The model under review builds one solid part; all positions refer to its coordinate system, in mm. A direction names the side the tool comes from. Give positions to 0.01 mm unless a question says otherwise; leave off trailing zeros. Order: outer loops, then holes, each group sorted by start corner. A loop starts at its lowest first (then second) coordinate and runs counter-clockwise, first axis right, second up.
```python
from build123d import *

# Parameters (mm, degrees)
BOSS_EXTRUDE1_DEPTH     = 19.05
CUT_EXTRUDE1_DEPTH      = 1
CUT_EXTRUDE1_DEPTH_BACK = 34.925
SKETCH4_R               = 2.794
CUT_EXTRUDE2_DEPTH      = 51.8
CUT_EXTRUDE2_DEPTH_BACK = 26.4
SKETCH5_R               = 2.794
CUT_EXTRUDE3_DEPTH      = 26.4
CUT_EXTRUDE3_DEPTH_BACK = 51.8
SKETCH6_R               = 2.794
CUT_EXTRUDE4_DEPTH      = 1
CUT_EXTRUDE4_DEPTH_BACK = 77.2
SKETCH7_R               = 6.35
CUT_EXTRUDE6_DEPTH      = 34.925


with BuildPart() as part:
    # Sketch1 → Boss-Extrude1 (new body, symmetric)
    with BuildSketch(Plane.YZ):
        with BuildLine():
            Line((6.35, 25.4), (67.818, 25.4))
            Line((67.818, 25.4), (67.818, 44.45))
            ThreePointArc((67.818, 44.45), (69.677871939, 48.940128061), (74.168, 50.8))
            Line((74.168, 50.8), (135.636, 50.8))
            Line((135.636, 50.8), (135.636, 69.85))
            ThreePointArc((135.636, 69.85), (137.495871939, 74.340128061), (141.986, 76.2))
            Line((141.986, 76.2), (203.454, 76.2))
            Line((203.454, 76.2), (203.454, 0))
            Line((203.454, 0), (112.272540658, 0))
            Line((112.272540658, 0), (108.743815039, 0))
            Line((108.743815039, 0), (0, 0))
            Line((0, 0), (0, 19.05))
            ThreePointArc((0, 19.05), (1.859871939, 23.540128061), (6.35, 25.4))
        make_face()
    extrude(amount=BOSS_EXTRUDE1_DEPTH, both=True)

    # Sketch2 → Cut-Extrude1 (cut, two sides)
    with BuildSketch(Plane.YZ.offset(19.05)) as cut_extrude1_sk:
        with BuildLine():
            Line((6.35, 22.225), (64.643, 22.225))
            Line((64.643, 22.225), (64.643, 3.175))
            Line((64.643, 3.175), (3.175, 3.175))
            Line((3.175, 3.175), (3.175, 19.05))
            ThreePointArc((3.175, 19.05), (4.10493597, 21.29506403), (6.35, 22.225))
        make_face()
        with BuildLine():
            Line((74.168, 47.625), (132.461, 47.625))
            Line((132.461, 47.625), (132.461, 3.175))
            Line((132.461, 3.175), (70.993, 3.175))
            Line((70.993, 3.175), (70.993, 44.45))
            ThreePointArc((70.993, 44.45), (71.92293597, 46.69506403), (74.168, 47.625))
        make_face()
        with BuildLine():
            Line((141.986, 73.025), (200.279, 73.025))
            Line((200.279, 73.025), (200.279, 3.175))
            Line((200.279, 3.175), (138.811, 3.175))
            Line((138.811, 3.175), (138.811, 69.85))
            ThreePointArc((138.811, 69.85), (139.74093597, 72.09506403), (141.986, 73.025))
        make_face()
    extrude(amount=CUT_EXTRUDE1_DEPTH, mode=Mode.SUBTRACT)
    extrude(cut_extrude1_sk.sketch, amount=-CUT_EXTRUDE1_DEPTH_BACK, mode=Mode.SUBTRACT)

    # Sketch4 → Cut-Extrude2 (cut, two sides)
    with BuildSketch(Plane.XY.offset(25.4)) as cut_extrude2_sk:
        with Locations((0, 17.78)):
            Circle(SKETCH4_R)
        with Locations((0, 49.53)):
            Circle(SKETCH4_R)
    extrude(amount=CUT_EXTRUDE2_DEPTH, mode=Mode.SUBTRACT)
    extrude(cut_extrude2_sk.sketch, amount=-CUT_EXTRUDE2_DEPTH_BACK, mode=Mode.SUBTRACT)

    # Sketch5 → Cut-Extrude3 (cut, two sides)
    with BuildSketch(Plane.XY.offset(50.8)) as cut_extrude3_sk:
        with Locations((0, 85.725)):
            Circle(SKETCH5_R)
        with Locations((0, 117.475)):
            Circle(SKETCH5_R)
    extrude(amount=CUT_EXTRUDE3_DEPTH, mode=Mode.SUBTRACT)
    extrude(cut_extrude3_sk.sketch, amount=-CUT_EXTRUDE3_DEPTH_BACK, mode=Mode.SUBTRACT)

    # Sketch6 → Cut-Extrude4 (cut, two sides)
    with BuildSketch(Plane.XY.offset(76.2)) as cut_extrude4_sk:
        with Locations((0, 156.21)):
            Circle(SKETCH6_R)
        with Locations((0, 187.96)):
            Circle(SKETCH6_R)
    extrude(amount=CUT_EXTRUDE4_DEPTH, mode=Mode.SUBTRACT)
    extrude(cut_extrude4_sk.sketch, amount=-CUT_EXTRUDE4_DEPTH_BACK, mode=Mode.SUBTRACT)

    # Sketch7 → Cut-Extrude6 (cut)
    with BuildSketch(Plane.XY.offset(3.175)):
        with Locations((0, 17.78)):
            Circle(SKETCH7_R)
        with Locations((0, 49.53)):
            Circle(SKETCH7_R)
        with Locations((0, 85.725)):
            Circle(SKETCH7_R)
        with Locations((0, 117.475)):
            Circle(SKETCH7_R)
        with Locations((0, 156.21)):
            Circle(SKETCH7_R)
        with Locations((0, 187.96)):
            Circle(SKETCH7_R)
    extrude(amount=-CUT_EXTRUDE6_DEPTH, mode=Mode.SUBTRACT)


solid = part.part
```
Item 1: For faces 1 (the flat face through (2, 103, 47.625)), 2 (the flat face through (19.05, 102, 50)), 3 (the flat face through (0, 135.636, 60)), list the 3-axis set-ups (+Z, -Z, +X, -X, +Y, -Y) from which the entire face can be reached by the end or side of a thin tool; tool diameter is ignored.
Values found:
face 1: +X
face 2: +Z, -Z, +X, +Y, -Y
face 3: +Z, +X, -X, -Y
Item 2: Draft analysis for pull direction X (two halves, no side actions). For faces 4 (the flat face through (-15.875, 34, 13)), 5 (the flat face through (0, 203.454, 39)), 6 (the cylindrical face through (-0.83, 92.02, 1.61)), state which applies: released by +X, released by -X, zero draft, split by the parting line, or undercut.
Values found:
face 4: released by +X
face 5: zero draft
face 6: undercut
Item 3: Take a section at D-D (y = 101). Give the boundary of the cut face in (x, z) (3 decimals), and give its area (3 significant figures).
Values found:
outline: (-19.05, 0) - (19.05, 0) - (19.05, 3.175) - (-15.875, 3.175) - (-15.875, 47.625) - (19.05, 47.625) - (19.05, 50.8) - (-19.05, 50.8) - close
area: 383 mm2
Item 4: For line 1 (Y direction, x = 3, z = 7.5) (3 decimals); line 2 (Y direction, x = -6.5, z = 30.5); line 3 (Y direction, x = 5.5, z = 59), list the stretches that pass through material, from the lowest coordinate up.
Values found:
line 1: y = 0 to 3.175, 64.643 to 70.993, 132.461 to 138.811, 200.279 to 203.454
line 2: y = 67.82 to 70.99, 132.46 to 138.81, 200.28 to 203.45
line 3: y = 135.64 to 138.81, 200.28 to 203.45
Item 5: Take a section at B-B (z = 31). Give the boundary of the cut face in (x, y) (3 decimals).
Values found:
outline: (-19.05, 67.818) - (19.05, 67.818) - (19.05, 70.993) - (-15.875, 70.993) - (-15.875, 132.461) - (19.05, 132.461) - (19.05, 138.811) - (-15.875, 138.811) - (-15.875, 200.279) - (19.05, 200.279) - (19.05, 203.454) - (-19.05, 203.454) - close
Item 6: Take a section at A-A (y = 187.96). Give the boundary of the cut face in (x, z) (3 decimals), and give its area (3 significant figures).
Values found:
outline: (-19.05, 0) - (-6.35, 0) - (-6.35, 3.175) - (-15.875, 3.175) - (-15.875, 73.025) - (-2.794, 73.025) - (-2.794, 76.2) - (-19.05, 76.2) - close; (2.794, 73.025) - (19.05, 73.025) - (19.05, 76.2) - (2.794, 76.2) - close; (6.35, 0) - (19.05, 0) - (19.05, 3.175) - (6.35, 3.175) - close
area: 406 mm2
Item 7: Take a section at C-C (x = -9). Give the boundary of the cut face in (y, z) (3 decimals).
Values found:
outline: (0, 0) - (203.454, 0) - (203.454, 76.2) - (141.986, 76.2) arc R6.35 ccw to (135.636, 69.85) - (135.636, 50.8) - (74.168, 50.8) arc R6.35 ccw to (67.818, 44.45) - (67.818, 25.4) - (6.35, 25.4) arc R6.35 ccw to (0, 19.05) - close; hole (3.175, 3.175) - (64.643, 3.175) - (64.643, 22.225) - (6.35, 22.225) arc R3.175 ccw to (3.175, 19.05) - close; hole (70.993, 3.175) - (132.461, 3.175) - (132.461, 47.625) - (74.168, 47.625) arc R3.175 ccw to (70.993, 44.45) - close; hole (138.811, 3.175) - (200.279, 3.175) - (200.279, 73.025) - (141.986, 73.025) arc R3.175 ccw to (138.811, 69.85) - close
Item 8: Clearance check with flat-ended pins moving along their axes: pin 1 Ø3.5 at (x, y) = (0, 17.78) entering from +Z; pin 2 Ø17.5 at (x, z) = (-2.5, 32.5) entering from -Y; pin 3 Ø21 at (x, z) = (-7, 63.5) entering from -Y; pin 4 Ø11.5 at (x, y) = (-8, 52) entering from +Z. State where each tip first meets the part, or that it passes through.
Values found:
pin 1: passes through
pin 2: stops at y = 2.08
pin 3: stops at y = 135.64
pin 4: stops at z = 25.4
